from build123d import *

# Parameters (mm, degrees)
F0_R     = 12.7
F1_DEPTH = 69.85
F2_D     = 6.5278
F3_R     = 3.2639
F4_DEPTH = 50.8
F5_R     = 3.175
F6_DEPTH = 12.7
F8_DEPTH = 12.7


with BuildPart() as f1:
    # F0 (on Front) → F1 (new body)
    with BuildSketch(Plane.XZ):
        Circle(F0_R)
    extrude(amount=F1_DEPTH)

    # F2 (through all)
    with Locations(Plane(origin=(0, 0, 0), x_dir=(1, 0, 0), z_dir=(0, 1, 0))):
        with Locations((0, 0)):
            Hole(F2_D / 2)

    # F3 (on face) → F4 (cut)
    with BuildSketch(Plane.XZ.offset(69.85)):
        with BuildLine():
            ThreePointArc((0, 12.7), (-1.7567894036, 12.5779048729), (-3.4798, 12.2139670853))
            Line((-3.4798, 12.2139670853), (-3.4798, -12.2139670853))
            ThreePointArc((-3.4798, -12.2139670853), (-1.7567894036, -12.5779048729), (0, -12.7))
            ThreePointArc((0, -12.7), (1.7567894036, -12.5779048729), (3.4798, -12.2139670853))
            Line((3.4798, -12.2139670853), (3.4798, 12.2139670853))
            ThreePointArc((3.4798, 12.2139670853), (1.7567894036, 12.5779048729), (0, 12.7))
        make_face()
        Circle(F3_R, mode=Mode.SUBTRACT)
    extrude(amount=-F4_DEPTH, mode=Mode.SUBTRACT)

    # F5 (on Right) → F6 (cut, symmetric)
    with BuildSketch(Plane.YZ):
        with Locations((-60.325, 0)):
            Circle(F5_R)
    extrude(amount=F6_DEPTH, both=True, mode=Mode.SUBTRACT)

    # F7 (on Right) → F8 (cut, symmetric)
    with BuildSketch(Plane.YZ):
        with BuildLine():
            Line((-34.925, 3.2131049847), (-50.8, 3.2131049847))
            ThreePointArc((-50.8, 3.2131049847), (-53.975, 0.0381049847), (-50.8, -3.1368950153))
            Line((-50.8, -3.1368950153), (-34.925, -3.1368950153))
            ThreePointArc((-34.925, -3.1368950153), (-31.75, 0.0381049847), (-34.925, 3.2131049847))
        make_face()
    extrude(amount=F8_DEPTH, both=True, mode=Mode.SUBTRACT)


solid = f1.part
Can you work these out from the model? Positions are in its coordinate system, mm. A direction names the side the tool comes from. Round coordinates to 2 decimals unless told otherwise and drop trailing zeros. Order: outer loops, then holes, each group sorted by start corner. A loop starts at its lowest first (then second) coordinate and runs counter-clockwise, first axis right, second up. Notation, with made-up numbers: (64.5, 19) - (119.5, 19) arc R19 cw to (119.5, 35) - close; hole circle Ø10 at (62.5, 28). An arc over 180 degrees is marked (long way). Answer in a Markdown table with one row per item.
(1) Suppose I cut it at A-A, the plane x = 0. Please give me the cut outline in (y, z).
From the geometry:
| item | result |
|---|---|
| outline | (-19.05, -12.7) - (0, -12.7) - (0, -3.26) - (-19.05, -3.26) - close; (-19.05, 3.26) - (0, 3.26) - (0, 12.7) - (-19.05, 12.7) - close |
(2) Which directions (+Z, -Z, +X, -X, +Y, -Y) give clear straight access to the entire face, cutting with the end or side of a thin tool? Please do faces 1 (the face through (7, -69.85, 0)), 2 (the face through (-8, -43, 3.213)), 3 (the face through (-3.48, -45, 6)).
From the geometry:
| item | result |
|---|---|
| face 1 | +Z, -Z, +X, -X, -Y |
| face 2 | +X, -X |
| face 3 | +Z, -Z, -Y |
(3) For P1, Ø3, axis at y = -23.5, z = 4, coming from the -X side; P2, Ø7, axis at x = 9, y = -39.5, coming from the -Z side; P3, Ø3, axis at y = -46, z = 3.5, coming from the +X side, each with a flat end and sliding along its axis, tell me the tip position at first contact or that it passes through.
From the geometry:
| item | result |
|---|---|
| P1 | stops at x = -12.45 |
| P2 | stops at z = -11.45 |
| P3 | stops at x = 12.29 |
(4) Suppose I cut it at B-B, the plane y = -39. Please give me the cut outline in (x, z), plus the area to 3 significant figures.
From the geometry:
| item | result |
|---|---|
| outline | (-12.31, -3.14) arc R12.7 ccw to (-3.48, -12.21) - (-3.48, -3.14) - close; (-12.29, 3.21) - (-3.48, 3.21) - (-3.48, 12.21) arc R12.7 ccw to start; (3.48, -12.21) arc R12.7 ccw to (12.31, -3.14) - (3.48, -3.14) - close; (3.48, 3.21) - (12.29, 3.21) arc R12.7 ccw to (3.48, 12.21) - close |
| area | 217 mm2 |
(5) If we mould it in two halves opening along Z, with no side actions, what happens to faces 4 (the face through (3, 0, -3)), 5 (the face through (-8.026, -53.974, 0.108)), 6 (the face through (12.114, -34.436, 3.815))? For each: released by +Z, released by -Z, zero draft, split by the parting line, or undercut.
From the geometry:
| item | result |
|---|---|
| face 4 | zero draft |
| face 5 | undercut |
| face 6 | split by the parting line |
(6) Suppose I cut it at C-C, the plane z = 0.75. Please give me the cut outline in (x, y), plus the area to 3 significant figures.
From the geometry:
| item | result |
|---|---|
| outline | (-12.68, -69.85) - (-3.48, -69.85) - (-3.48, -63.41) - (-12.68, -63.41) - close; (-12.68, -57.24) - (-3.48, -57.24) - (-3.48, -53.89) - (-12.68, -53.89) - close; (-12.68, -31.83) - (-3.48, -31.83) - (-3.48, -19.05) - (-3.18, -19.05) - (-3.18, 0) - (-12.68, 0) - close; (3.18, -19.05) - (3.48, -19.05) - (3.48, -31.83) - (12.68, -31.83) - (12.68, 0) - (3.18, 0) - close; (3.48, -69.85) - (12.68, -69.85) - (12.68, -63.41) - (3.48, -63.41) - close; (3.48, -57.24) - (12.68, -57.24) - (12.68, -53.89) - (3.48, -53.89) - close |
| area | 777 mm2 |
(7) Suppose I cut it at D-D, the plane y = -65. Please give me the cut outline in (x, z).
From the geometry:
| item | result |
|---|---|
| outline | (-3.48, -12.21) - (-3.48, 12.21) arc R12.7 ccw to start; (3.48, -12.21) arc R12.7 ccw to (3.48, 12.21) - close |
(8) Please list where these lines run through material, in increasing order: L1, parallel to X at y = -38.5, z = 3.5; L2, parallel to X at y = -11, z = 0; L3, parallel to Z at x = 5.75, y = -36. Write a range as from..to.
From the geometry:
| item | result |
|---|---|
| L1 | x = -12.21..-3.48, 3.48..12.21 |
| L2 | x = -12.7..-3.26, 3.26..12.7 |
| L3 | z = -11.32..-3.14, 3.21..11.32 |
